Source: CAD feature listing. Evaluate the final solid. Frame: model axes, mm. A direction names the side the tool comes from. Coordinates: 2 decimals unless noted, no trailing zeros. Order: outer loops, then holes, each group sorted by start corner. A loop starts at its lowest first (then second) coordinate and runs counter-clockwise, first axis right, second up.
```python
from build123d import *

# Parameters (mm, degrees)
SKETCH_2_R          = 3
CUT_EXTRUDE_3_DEPTH = 35
CUT_EXTRUDE_START   = -10
SKETCH_4_R          = 6
CUT_EXTRUDE_4_DEPTH = 52


with BuildPart() as part:
    # Эскиз1 → Повернуть2 (revolve)
    with BuildSketch(Plane.XY, mode=Mode.PRIVATE) as revolve_2_sk:
        Polygon((30, 0), (32.500012812, 0), (32.679297783, 56), (56.5, 103), (56.5, 106), (32.5, 106), (32.5, 102), (30.159832694, 49.92404441), align=None)
    revolve(revolve_2_sk.sketch.rotate(Axis((0, 0, 0), (0, 1, 0)), 90), axis=Axis((0, 0, 0), (0, 1, 0)))

    # Эскиз2 → Вырез-Вытянуть3 (cut)
    with BuildSketch(Plane(origin=(0, 106, 0), x_dir=(1, 0, 0), z_dir=(0, 1, 0))):
        with Locations(Location((-39.5, 0, 0), (0, 0, 270))):
            Circle(SKETCH_2_R)
    cut_extrude_3 = extrude(amount=-CUT_EXTRUDE_3_DEPTH, mode=Mode.SUBTRACT)

    # Зеркальное отражение1: Вырез-Вытянуть3 across plane
    add(cut_extrude_3.mirror(Plane(origin=(0, 0, 0), x_dir=(0, 0, 1), z_dir=(1, 0, 0))), mode=Mode.SUBTRACT)

    # Эскиз4 → Вырез-Вытянуть4 (cut)
    with BuildSketch(Plane(origin=(0, 56, 0), x_dir=(1, 0, 0), z_dir=(0, 1, 0)).offset(CUT_EXTRUDE_START)):
        with Locations(Location((39.5, 0, 0), (0, 0, 270))):
            Circle(SKETCH_4_R)
    cut_extrude_4 = extrude(amount=CUT_EXTRUDE_4_DEPTH, mode=Mode.SUBTRACT)

    # Зеркальное отражение2: Вырез-Вытянуть4 across plane
    add(cut_extrude_4.mirror(Plane(origin=(0, 0, 0), x_dir=(0, 0, 1), z_dir=(1, 0, 0))), mode=Mode.SUBTRACT)


solid = part.part
```
1. Draft query along Z for faces 4 (the cylindrical face through (-9.76, 103.97, -31)), 5 (the flat face through (9, 0, 29)), 6 (the conical face through (35.94, 64.16, 7.98)). Return one class per face: +Z half, -Z half, draft (parallel to the pull), parting line (faces both ways), or undercut.
2. Section query C-C, the plane y = 87. Output: boundary loops of the cut face in (x, z), plus the area to 3 significant figures.
3. Contact query for flat-ended pins moving along their axis: P1, Ø3.5, axis at x = 37.5, z = 1, coming from the -Y side; P2, Ø5, axis at x = -39.5, z = 0, coming from the +Y side; P3, Ø4, axis at y = 76, z = -17, coming from the +X side; P4, Ø3, axis at y = 12, z = -8.5, coming from the -X side. Output: stop coordinate, or through.
4. Section query D-D, the plane y = 41. Output: boundary loops of the cut face in (x, z), plus the area to 3 significant figures.
5. Section query B-B, the plane z = 1. Count the separate pieces of the cut face and the enclosed holes in it, plus the area to 3 significant figures.
6. Section query A-A, the plane y = 74.5. Output: boundary loops of the cut face in (x, z), plus the area to 3 significant figures.
7. Access query for faces 1 (the conical face through (29.364, 24.613, 6.52)), 2 (the cylindrical face through (36.97, 102.06, 1.61)), 3 (the flat face through (-38, 98, -3)). Directions: +Z, -Z, +X, -X, +Y, -Y. A direction counts if a zero-diameter tool reaches every point of the face in a straight line with its end or side. Return the directions, or none.
8. Material intervals for line 1 along X through (y, z) = (103, 0); line 2 along X through (y, z) = (100.75, 0); line 3 along X through (y, z) = (76, 0), sorted ascending.
Answer key:
1. face 4: undercut
1. face 5: draft
1. face 6: parting line
2. outline: circle Ø96.78 at (0, 0); hole circle Ø12 at (-39.5, 0); hole circle Ø63.65 at (0, 0); hole circle Ø12 at (39.5, 0)
2. area: 3,950 mm2
3. P1: stops at y = 98
3. P2: passes through
3. P3: stops at x = 40.67
3. P4: stops at x = -31.78
4. outline: circle Ø65.26 at (0, 0); hole circle Ø60.26 at (0, 0)
4. area: 493 mm2
5. separate pieces: 4
5. enclosed holes: 0
5. area: 889 mm2
6. outline: (-41.68, -5.59) arc R42.06 ccw to (41.68, -5.59) arc R6 cw (long way) to (41.68, 5.59) arc R42.06 ccw to (-41.68, 5.59) arc R6 cw (long way) to start; hole circle Ø62.53 at (0, 0)
6. area: 2,320 mm2
7. face 1: +Y
7. face 2: +Y, -Y
7. face 3: -Y
8. line 1: x = -56.5 to -42.5, -36.5 to -32.5, 32.5 to 36.5, 42.5 to 56.5
8. line 2: x = -55.36 to -42.5, -36.5 to -32.44, 32.44 to 36.5, 42.5 to 55.36
8. line 3: x = -33.5 to -31.33, 31.33 to 33.5
